Check sheet for the modelled part. Datum: model origin and axes. Units: mm. A direction names the side the tool comes from. Round coordinates to 2 decimals unless told otherwise and drop trailing zeros. Order: outer loops, then holes, each group sorted by start corner. A loop starts at its lowest first (then second) coordinate and runs counter-clockwise, first axis right, second up.
Q1. Cross-section at C-C on x = 107. Record the cut outline in (y, z) (3 decimals).
Q2. Scan lines: probe 1 along X at (y, z) = (-5.5, -15.75); probe 2 along Z at (x, y) = (27, -11.5) (3 decimals); probe 3 along X at (y, z) = (-8.75, -4). Record each from-to range of solid material in increasing order.
Q3. Mould release check, pull along X, two halves, no side actions. Record for faces 1 (the flat face through (65, -2, -28.732)), 2 (the flat face through (19, -7, -5.1)), 3 (the flat face through (0, -5, -11)): +X half, -X half, draft (parallel to the pull), parting line (faces both ways), or undercut.
Q4. Cross-section at B-B on z = -14. Record the cut outline in (x, y), then the cut area to 3 significant figures.
Q5. Set-up check for faces 4 (the flat face through (34, 0, -5)), 5 (the cylindrical face through (2.9, -2.72, -22.72)), 6 (the flat face through (26.95, -7.3, -2.51)): record each of +Z, -Z, +X, -X, +Y, -Y from which the full face is reachable in a straight line by a thin tool's end or side.
Q6. Depth check by flat-ended pin: P1, Ø8, axis at x = 35.5, y = -12.5, coming from the -Z side (3 decimals); P2, Ø4.5, axis at y = -5.5, z = -15.5, coming from the +X side; P3, Ø3, axis at x = 92, z = -3.5, coming from the +Y side; P4, Ø1, axis at y = -9, z = -23, coming from the +X side. Enter the tip coordinate at first touch or a pass-through.
Q7. Cross-section at A-A on y = -9.5. Give the number of separate pieces and of enclosed holes in the cut face, then the cut area to 3 significant figures.
from build123d import *

# Parameters (mm, degrees)
EXTRUDE2_DEPTH                 = 143.3725
BOSS_EXTRUDE4_DEPTH            = 6.35
BOSS_EXTRUDE5_DEPTH            = 6.35
M3X0_5_TAPPED_HOLE1_D          = 3
M3X0_5_TAPPED_HOLE1_DEPTH      = 7.5
M3X0_5_TAPPED_HOLE1_TIP        = 0.901290929
F_2_5_2_5_DIAMETER_HOLE1_D     = 2.5
F_2_5_2_5_DIAMETER_HOLE1_DEPTH = 6.35
F_2_5_2_5_DIAMETER_HOLE1_TIP   = 0.751075774
CUT_EXTRUDE1_DEPTH             = 5.1
F_4_CLEARANCE_HOLE1_D          = 2.9464


with BuildPart() as part:
    # Sketch73 → Extrude2 (new body)
    with BuildSketch(Plane(origin=(0, 0, 0), x_dir=(0, 0, -1), z_dir=(1, 0, 0))):
        Polygon((0, 0), (10.525, 0), (10.525, -14.62), (0, -14.18), align=None)
    extrude(amount=EXTRUDE2_DEPTH)

    # Sketch113 → Boss-Extrude4 (add)
    with BuildSketch(Plane.ZY):
        Polygon((-28.732, 0.5), (0, 0.5), (0, -14.18), (-10.525, -14.62), (-28.732, -4.108183649), align=None)
    extrude(amount=-BOSS_EXTRUDE4_DEPTH)

    # Sketch114 → Boss-Extrude5 (add)
    with BuildSketch(Plane.ZY.offset(-62.1372)):
        Polygon((-10.525, -14.62), (-10.525, 0), (0, 0), (0, 0.5), (-28.732, 0.5), (-28.732, -4.108183649), align=None)
    extrude(amount=-BOSS_EXTRUDE5_DEPTH)

    # M3x0.5 Tapped Hole1
    with Locations(Plane(origin=(-41.488675912, 0.5, -11.380370452), x_dir=(-1, 0, 0), z_dir=(0, 1, 0))):
        with Locations((-106.800875912, 0.880370452), (-44.663675912, 0.880370452)):
            Hole(M3X0_5_TAPPED_HOLE1_D / 2, depth=M3X0_5_TAPPED_HOLE1_DEPTH)
            with Locations((0, 0, -(M3X0_5_TAPPED_HOLE1_DEPTH + M3X0_5_TAPPED_HOLE1_TIP / 2))):  # 118° drill point
                Cone(0, M3X0_5_TAPPED_HOLE1_D / 2, M3X0_5_TAPPED_HOLE1_TIP, mode=Mode.SUBTRACT)

    # 2.5 _2.5_ Diameter Hole1
    with Locations(Plane(origin=(0, 0.5, 0), x_dir=(-1, 0, 0), z_dir=(0, 1, 0))):
        with Locations((-3.175, -21.5), (-65.3122, -21.5)):
            Hole(F_2_5_2_5_DIAMETER_HOLE1_D / 2, depth=F_2_5_2_5_DIAMETER_HOLE1_DEPTH)
            with Locations((0, 0, -(F_2_5_2_5_DIAMETER_HOLE1_DEPTH + F_2_5_2_5_DIAMETER_HOLE1_TIP / 2))):  # 118° drill point
                Cone(0, F_2_5_2_5_DIAMETER_HOLE1_D / 2, F_2_5_2_5_DIAMETER_HOLE1_TIP, mode=Mode.SUBTRACT)

    # Sketch117 → Cut-Extrude1 (cut)
    with BuildSketch(Plane.XY):
        Polygon((30.967580189, 0), (14.483, 0), (6.432290426, -14.62), (22.916870615, -14.62), align=None)
    extrude(amount=-CUT_EXTRUDE1_DEPTH, mode=Mode.SUBTRACT)

    # 4 Clearance Hole1 (through all)
    with Locations(Plane(origin=(0, 0, -10.525), x_dir=(-1, 0, 0), z_dir=(0, 0, -1))):
        with Locations((-119.4195, -3.5), (-119.4195, -9.5), (-49.4195, -3.5), (-49.4195, -9.5)):
            Hole(F_4_CLEARANCE_HOLE1_D / 2)


solid = part.part
Results found:
1. outline: (-14.62, -10.525) - (0, -10.525) - (0, 0) - (-14.18, 0) - close
2. probe 1: x = 0 to 6.35, 62.14 to 68.49
2. probe 2: z = -10.525 to 0
2. probe 3: x = 0 to 9.66, 26.15 to 48.15, 50.69 to 118.15, 120.69 to 143.37
3. face 1: draft
3. face 2: undercut
3. face 3: -X half
4. outline: (0, -12.61) - (6.35, -12.61) - (6.35, 0.5) - (0, 0.5) - close; (62.14, -12.61) - (68.49, -12.61) - (68.49, 0.5) - (62.14, 0.5) - close
4. area: 167 mm2
5. face 4: +Z, -Z, +Y
5. face 5: +Y
5. face 6: +Z, +Y
6. P1: stops at z = -10.525
6. P2: stops at x = 68.49
6. P3: stops at y = 0
6. P4: passes through
7. separate pieces: 3
7. enclosed holes: 0
7. area: 1,480 mm2
